Study the drawing (mm; zero at the part's minimum x, y, z) and answer. A direction names the side the tool comes from. Round coordinates to 2 decimals unless told otherwise and drop trailing zeros. Write each loop counter-clockwise with the first axis right and the second up, starting at its lowest first coordinate (ties: lowest second). Pieces come first, ordered by that corner, then holes.
(1) A cutting plane is placed at B-B, the plane y = 50. Give the vertices of the cut face in (x, z).
(2) Each of these flat-tipped pins is pushed along its axis until it touches: pin 1 Ø3 at (x, y) = (13.5, 83) entering from -Z; pin 2 Ø15 at (x, y) = (32, 54.5) entering from -Z; pin 3 Ø20 at (x, y) = (6.5, 45.5) entering from +Z. Where does it stop, or does it pass through?
(3) For the marked faces 4, 5, 6 and 7, determine the directions among +Z, -Z, +X, -X, +Y, -Y from which every point of the face is accessible in a straight line to the end or side of a thin tool.
(4) The mould has two halves that part along Y. Classify the marked faces 1, 2 and 3: +Y half, -Y half, draft (parallel to the pull), parting line (faces both ways), or undercut.
(5) A cutting plane is placed at A-A, the plane z = 170. Give the vertices of the cut face in (x, y).
(6) A cutting plane is placed at D-D, the plane z = 249. Give the vertices of the cut face in (x, y).
(7) A cutting plane is placed at C-C, the plane x = 17.5. Give the vertices of the cut face in (y, z), and give its area (3 significant figures).
(8) Find the intervals of material crossed by probe 1 along Z at (x, y) = (38.75, 50); probe 2 along Z at (x, y) = (43, 50); probe 3 along X at (y, z) = (50.5, 22), in increasing order.
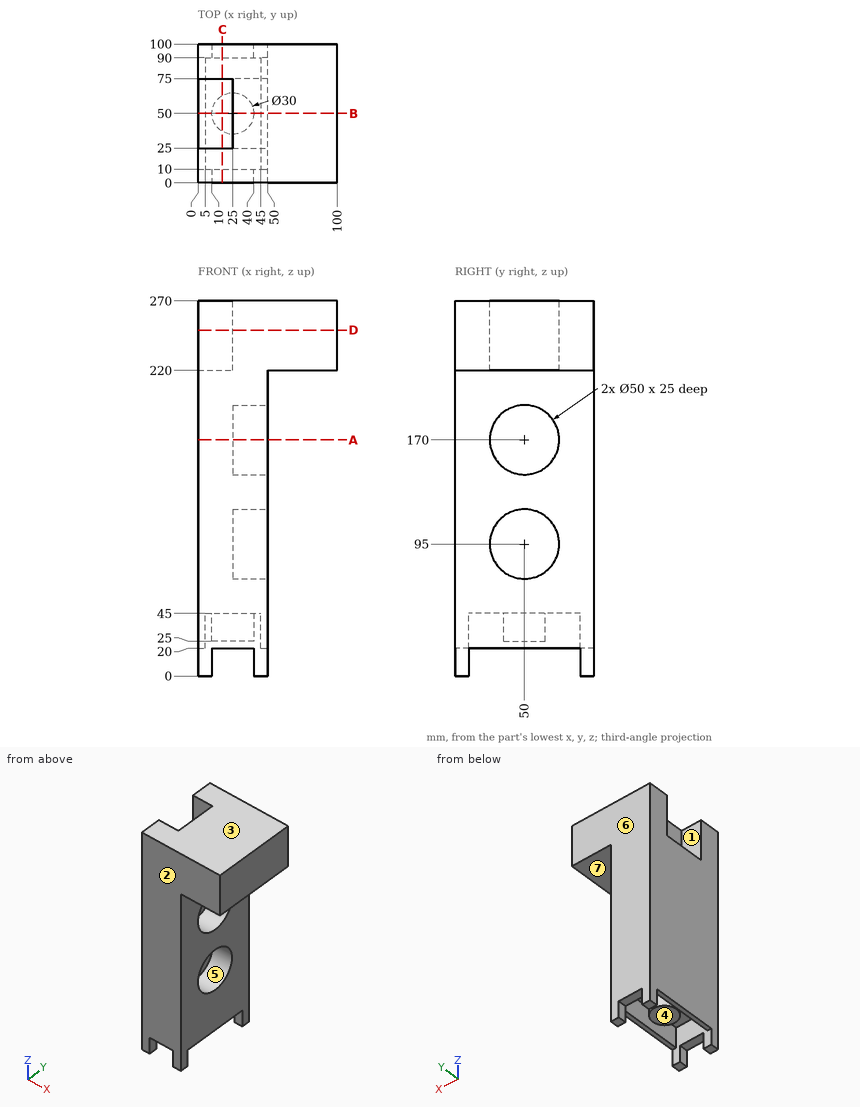
Solutions:
1. outline: (0, 20) - (5, 20) - (5, 45) - (10, 45) - (10, 25) - (40, 25) - (40, 45) - (45, 45) - (45, 20) - (50, 20) - (50, 70) - (25, 70) - (25, 120) - (50, 120) - (50, 145) - (25, 145) - (25, 195) - (50, 195) - (50, 220) - (100, 220) - (100, 270) - (25, 270) - (25, 220) - (0, 220) - close
2. pin 1: stops at z = 45
2. pin 2: stops at z = 25
2. pin 3: stops at z = 220
3. face 4: -Z
3. face 5: +X
3. face 6: +Z, -Z, +X, -X, +Y
3. face 7: -Z, +X, +Y, -Y
4. face 1: undercut
4. face 2: -Y half
4. face 3: draft
5. outline: (0, 0) - (50, 0) - (50, 25) - (25, 25) - (25, 75) - (50, 75) - (50, 100) - (0, 100) - close
6. outline: (0, 0) - (100, 0) - (100, 100) - (0, 100) - (0, 75) - (25, 75) - (25, 25) - (0, 25) - close
7. outline: (0, 20) - (10, 20) - (10, 45) - (37.01, 45) - (37.01, 25) - (62.99, 25) - (62.99, 45) - (90, 45) - (90, 20) - (100, 20) - (100, 270) - (75, 270) - (75, 220) - (25, 220) - (25, 270) - (0, 270) - close
7. area: 21,000 mm2
8. probe 1: z = 25 to 70, 120 to 145, 195 to 270
8. probe 2: z = 45 to 70, 120 to 145, 195 to 270
8. probe 3: x = 0 to 5, 45 to 50
